Work out the finished part from the listing and answer in its coordinate system (mm). Face numbers are marked on the shaded views. A direction names the side the tool comes from. Give positions to 0.01 mm unless a question says otherwise; leave off trailing zeros. Write each loop counter-clockwise with the first axis right and the second up, starting at its lowest first coordinate (ties: lowest second). Pieces come first, ordered by that corner, then holes. Notation, with made-up numbers: (-18.75, 72) - (23.25, 72) arc R18 ccw to (23.25, 82) - close; hole circle Ø3 at (-20, -3.5). An arc over 180 degrees is marked (long way). Write each question's results on one line, items separated by ' | '. Start each with the question number.
from build123d import *

# Parameters (mm, degrees)
SKETCH2_W           = 101.6
SKETCH2_H           = 101.6
BOSS_EXTRUDE2_DEPTH = 5
SKETCH3_W           = 5
SKETCH3_H           = 50.8
BOSS_EXTRUDE3_DEPTH = 25.4
SKETCH4_W           = 5
SKETCH4_H           = 50.8
BOSS_EXTRUDE4_DEPTH = 25.4
SKETCH8_R           = 3.556
CUT_EXTRUDE1_DEPTH  = 135.392047756
CUT_EXTRUDE2_REACH  = 136.392
SKETCH9_R           = 0.762
SKETCH11_R          = 7.9502
CUT_EXTRUDE3_DEPTH  = 146.911891222
CUT_EXTRUDE5_REACH  = 136.392
SKETCH18_R          = 0.762
SKETCH19_W          = 22.350467385
SKETCH19_H          = 21.198381437
BOSS_EXTRUDE5_DEPTH = 76.2
SKETCH22_R          = 7.94
CUT_EXTRUDE7_DEPTH  = 72.2
SKETCH23_R          = 4.95
CUT_EXTRUDE8_DEPTH  = 179.909697893


with BuildPart() as part:
    # Sketch2 → Boss-Extrude2 (new body)
    with BuildSketch(Plane(origin=(0, 0, 0), x_dir=(1, 0, 0), z_dir=(0, 1, 0))):
        with Locations((50.8, -50.8)):
            Rectangle(SKETCH2_W, SKETCH2_H)
    extrude(amount=BOSS_EXTRUDE2_DEPTH)

    # Sketch3 → Boss-Extrude3 (add)
    with BuildSketch(Plane(origin=(0, 5, 0), x_dir=(1, 0, 0), z_dir=(0, 1, 0))):
        with Locations((21.55, -50.8)):
            Rectangle(SKETCH3_W, SKETCH3_H)
    extrude(amount=BOSS_EXTRUDE3_DEPTH)

    # Sketch4 → Boss-Extrude4 (add)
    with BuildSketch(Plane(origin=(0, 5, 0), x_dir=(1, 0, 0), z_dir=(0, 1, 0))):
        with Locations((80.05, -50.8)):
            Rectangle(SKETCH4_W, SKETCH4_H)
    extrude(amount=BOSS_EXTRUDE4_DEPTH)

    # Sketch8 → Cut-Extrude1 (cut, through all)
    with BuildSketch(Plane.ZY.offset(-19.05)):
        with Locations((50.8, 23.542)):
            Circle(SKETCH8_R)
    extrude(amount=-CUT_EXTRUDE1_DEPTH, mode=Mode.SUBTRACT)

    # Sketch9 → Cut-Extrude2 (cut, up to next)
    with BuildSketch(Plane(origin=(82.55, 0, 0), x_dir=(0, 0, -1), z_dir=(1, 0, 0)), mode=Mode.PRIVATE) as cut_extrude2_sk1:
        with Locations((-50.8, 12.62)):
            Circle(SKETCH9_R)
    cut_extrude2_tool1 = extrude(cut_extrude2_sk1.sketch, amount=-CUT_EXTRUDE2_REACH, mode=Mode.PRIVATE) & part.part
    add(cut_extrude2_tool1.solids().sort_by_distance((82.55, 12.62, 50.8))[0], mode=Mode.SUBTRACT)

    # Sketch11 → Cut-Extrude3 (cut, through all)
    with BuildSketch(Plane(origin=(0, 5, 0), x_dir=(1, 0, 0), z_dir=(0, 1, 0))):
        with Locations(Location((59.61, -50.8, 0), (0, 0, 270))):
            Circle(SKETCH11_R)
    extrude(amount=-CUT_EXTRUDE3_DEPTH, mode=Mode.SUBTRACT)

    # Sketch18 → Cut-Extrude5 (cut, up to next)
    with BuildSketch(Plane.ZY.offset(-19.05), mode=Mode.PRIVATE) as cut_extrude5_sk1:
        with Locations(Location((50.8, 12.62, 0), (0, 0, 180))):
            Circle(SKETCH18_R)
    cut_extrude5_tool1 = extrude(cut_extrude5_sk1.sketch, amount=-CUT_EXTRUDE5_REACH, mode=Mode.PRIVATE) & part.part
    add(cut_extrude5_tool1.solids().sort_by_distance((19.05, 12.62, 50.8))[0], mode=Mode.SUBTRACT)

    # Sketch19 → Boss-Extrude5 (add)
    with BuildSketch(Plane.XZ):
        with Locations((59.324658632, 50.761526183)):
            Rectangle(SKETCH19_W, SKETCH19_H)
    extrude(amount=BOSS_EXTRUDE5_DEPTH)

    # Sketch22 → Cut-Extrude7 (cut)
    with BuildSketch(Plane(origin=(0, 0, 0), x_dir=(1, 0, 0), z_dir=(0, 1, 0))):
        with Locations(Location((59.61, -50.8, 0), (0, 0, 270))):
            Circle(SKETCH22_R)
    extrude(amount=-CUT_EXTRUDE7_DEPTH, mode=Mode.SUBTRACT)

    # Sketch23 → Cut-Extrude8 (cut, through all)
    with BuildSketch(Plane.XZ.offset(76.2)):
        with Locations(Location((59.61, 50.8, 0), (0, 0, 270))):
            Circle(SKETCH23_R)
    extrude(amount=-CUT_EXTRUDE8_DEPTH, mode=Mode.SUBTRACT)


solid = part.part
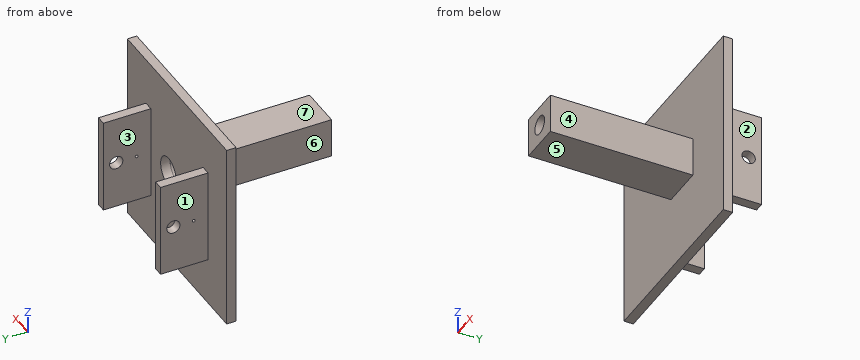
Q1. A tool of negligible diameter and unlimited length cuts with its end or side. For the marked faces 4, 5, 6 and 7, from which of +Z, -Z, +X, -X, +Y, -Y can it reach the whole face along a straight path? Write none if from no direction.
Q2. Consider L1, parallel to X at y = -73.25, z = 50.8; L2, parallel to X at y = 14.5, z = 63; L3, parallel to Z at x = 59, y = 2. Determine where each line is inside the solid, lowest interval first.
Q3. A cutting plane is placed at D-D, the plane z = 74. Write down the section's boundary in (x, y).
Q4. A cutting plane is placed at A-A, the plane y = 7. Write down the section's boundary in (x, z).
Q5. Given pin 1 (6.5 mm diameter, centred on y = -55.5, z = 46.5, fed in from -X); pin 2 (1.5 mm diameter, centred on y = -1.5, z = 81.5, fed in from -X); pin 3 (7.5 mm diameter, centred on y = 15, z = 61, fed in from +X); pin 4 (6 mm diameter, centred on x = 53, y = -43.5, fed in from -Z), each flat-ended and moving along its own axis, determine where each tip first touches the part or whether it passes through.
Q6. The mould has two halves that part along X. Classify the marked faces 1, 2 and 3: pulls with the +X half, pulls with the -X half, needs draft (parallel to the pull), parting line crosses it, or undercut.
Q7. A cutting plane is placed at C-C, the plane y = -50.5. Write down the section's boundary in (x, z).
Result:
1) face 4: +Z, -Z, +X, -Y | face 5: -Z, +X, -X, -Y | face 6: +Z, -Z, -X, -Y | face 7: +Z, +X, -X, -Y
2) L1: x = 48.15 to 54.66, 64.56 to 70.5 | L2: x = 19.05 to 24.05, 77.55 to 82.55 | L3: z = 0 to 42.87, 58.73 to 101.6
3) outline: (0, 0) - (101.6, 0) - (101.6, 5) - (82.55, 5) - (82.55, 30.4) - (77.55, 30.4) - (77.55, 5) - (24.05, 5) - (24.05, 30.4) - (19.05, 30.4) - (19.05, 5) - (0, 5) - close
4) outline: (19.05, 25.4) - (24.05, 25.4) - (24.05, 76.2) - (19.05, 76.2) - close; (77.55, 25.4) - (82.55, 25.4) - (82.55, 76.2) - (77.55, 76.2) - close
5) pin 1: stops at x = 48.15 | pin 2: passes through | pin 3: stops at x = 82.55 | pin 4: stops at z = 40.16
6) face 1: pulls with the -X half | face 2: pulls with the +X half | face 3: undercut
7) outline: (48.15, 40.16) - (70.5, 40.16) - (70.5, 61.36) - (48.15, 61.36) - close; hole circle Ø15.88 at (59.61, 50.8)
